from build123d import *

# Parameters (mm, degrees)
F0_W     = 78.115409
F0_H     = 12.533441
F1_DEPTH = 44.45
F3_DEPTH = 12.192
F5_DEPTH = 12.7


with BuildPart() as f1:
    # F0 (on Front) → F1 (new body)
    with BuildSketch(Plane.XZ):
        with Locations((-19.528851, 37.600327)):
            Rectangle(F0_W, F0_H)
    extrude(amount=F1_DEPTH)

    # F2 (on face) → F3 (join)
    with BuildSketch(Plane(origin=(0, 0, 31.333607), x_dir=(1, 0, 0), z_dir=(0, 0, -1))):
        Polygon((-25.35836, 0), (-38.474753, 44.45), (-58.586556, 44.45), (-58.586556, 0), align=None)
    extrude(amount=F3_DEPTH)

    # F4 (on face) → F5 (join)
    with BuildSketch(Plane(origin=(0, 0, 31.333607), x_dir=(1, 0, 0), z_dir=(0, 0, -1))):
        Polygon((4.372132, 44.45), (-5.829508, 0), (19.528853, 0), (19.528853, 44.45), align=None)
    extrude(amount=F5_DEPTH)


solid = f1.part
Part model, mm, in its own coordinate system. A direction names the side the tool comes from. Give positions to 0.01 mm unless a question says otherwise; leave off trailing zeros. Write each loop counter-clockwise with the first axis right and the second up, starting at its lowest first coordinate (ties: lowest second). Pieces come first, ordered by that corner, then holes.
1) Cut at B-B on y = -3. Write the cut outline in (x, z).
Resolved:
outline: (-58.59, 19.14) - (-26.24, 19.14) - (-26.24, 31.33) - (-5.14, 31.33) - (-5.14, 18.63) - (19.53, 18.63) - (19.53, 43.87) - (-58.59, 43.87) - close
2) Cut at A-A on z = 24. Write the cut outline in (x, y), then the cut area to 3 significant figures.
Resolved:
outline: (-58.59, -44.45) - (-38.47, -44.45) - (-25.36, 0) - (-58.59, 0) - close; (-5.83, 0) - (4.37, -44.45) - (19.53, -44.45) - (19.53, 0) - close
area: 2,090 mm2
3) Which spindle directions (+Z, -Z, +X, -X, +Y, -Y) get a long thin tool onto all of the face, cutting with end or side? Do faces 4 (the face through (-20, -22, 43.867)), 5 (the face through (-0.657, -22.536, 25.073)). Say none if no direction does.
Resolved:
face 4: +Z, +X, -X, +Y, -Y
face 5: -Z, -Y
4) Cut at C-C on x = -9. Write the cut outline in (y, z).
Resolved:
outline: (-44.45, 31.33) - (0, 31.33) - (0, 43.87) - (-44.45, 43.87) - close
5) Pin check, flat tips, straight feed: pin 1 (10 mm diameter, centred on x = -40.5, y = -31.5, fed in from -Z); pin 2 (13 mm diameter, centred on x = -13, y = -22.5, fed in from -Z). Stop position of each tip, or through.
Resolved:
pin 1: stops at z = 19.14
pin 2: stops at z = 31.33
6) Probe L1, parallel to X at y = -42, z = 29.25; L2, parallel to Z at x = -38.5, y = -34; L3, parallel to X at y = -41, z = 24.75. List the from-to ranges inside material, lowest first.
Resolved:
L1: x = -58.59 to -37.75, 3.81 to 19.53
L2: z = 19.14 to 43.87
L3: x = -58.59 to -37.46, 3.58 to 19.53
7) Two-plate mould, pull along X, no slides. Class faces 1 (the face through (-46, -23, 19.142)), 2 (the face through (-58.587, -22, 38)), 3 (the face through (-17, -27, 31.334)): released by +X, released by -X, zero draft, split by the parting line, or undercut.
Resolved:
face 1: zero draft
face 2: released by -X
face 3: undercut
8) Cut at D-D on y = -30.5. Write the cut outline in (x, z).
Resolved:
outline: (-58.59, 19.14) - (-34.36, 19.14) - (-34.36, 31.33) - (1.17, 31.33) - (1.17, 18.63) - (19.53, 18.63) - (19.53, 43.87) - (-58.59, 43.87) - close
